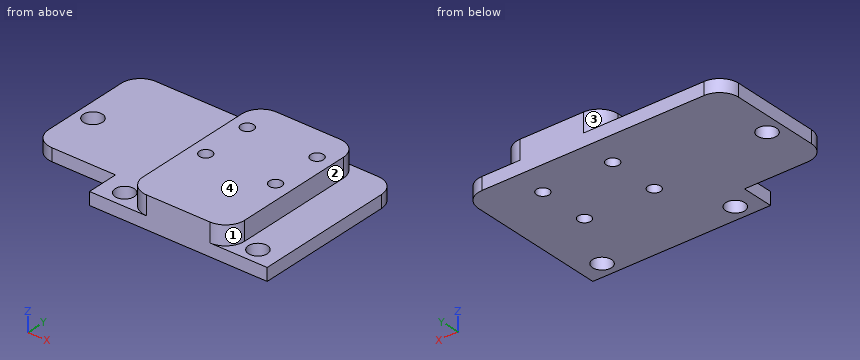
from build123d import *

# Parameters (mm, degrees)
BOSS_EXTRU_1_DEPTH      = 2
ESQUISSE2_W             = 16
ESQUISSE2_H             = 25
BOSS_EXTRU_2_DEPTH      = 3
ENL_V_MAT_EXTRU_1_REACH = 4
ESQUISSE3_R             = 1.5
ENL_V_MAT_EXTRU_2_REACH = 7
ESQUISSE4_R             = 1
ENL_V_MAT_EXTRU_3_REACH = 4
ESQUISSE5_W             = 13
ESQUISSE5_H             = 20
CONG_1_R                = 3


with BuildPart() as part:
    # Esquisse1 → Boss.-Extru.1 (new body)
    with BuildSketch(Plane.XY):
        Polygon((-27, 25), (27, 25), (27, 5), (14, 5), (14, 0), (-14, 0), (-14, 5), (-27, 5), align=None)
    extrude(amount=BOSS_EXTRU_1_DEPTH)

    # Esquisse2 → Boss.-Extru.2 (add)
    with BuildSketch(Plane.XY.offset(2)):
        with Locations((0, 12.5)):
            Rectangle(ESQUISSE2_W, ESQUISSE2_H)
    extrude(amount=BOSS_EXTRU_2_DEPTH)

    # Esquisse3 → Enlèv. mat.-Extru.1 (cut, up to next)
    with BuildSketch(Plane.XY.offset(2), mode=Mode.PRIVATE) as enl_v_mat_extru_1_sk1:
        with Locations((-24.5, 13.5)):
            Circle(ESQUISSE3_R)
    enl_v_mat_extru_1_tool1 = extrude(enl_v_mat_extru_1_sk1.sketch, amount=-ENL_V_MAT_EXTRU_1_REACH, mode=Mode.PRIVATE) & part.part
    add(enl_v_mat_extru_1_tool1.solids().sort_by_distance((-24.5, 13.5, 2))[0], mode=Mode.SUBTRACT)
    # Esquisse3 → Enlèv. mat.-Extru.1 (cut, up to next)
    with BuildSketch(Plane.XY.offset(2), mode=Mode.PRIVATE) as enl_v_mat_extru_1_sk2:
        with Locations((-10.5, 2.5)):
            Circle(ESQUISSE3_R)
    enl_v_mat_extru_1_tool2 = extrude(enl_v_mat_extru_1_sk2.sketch, amount=-ENL_V_MAT_EXTRU_1_REACH, mode=Mode.PRIVATE) & part.part
    add(enl_v_mat_extru_1_tool2.solids().sort_by_distance((-10.5, 2.5, 2))[0], mode=Mode.SUBTRACT)
    # Esquisse3 → Enlèv. mat.-Extru.1 (cut, up to next)
    with BuildSketch(Plane.XY.offset(2), mode=Mode.PRIVATE) as enl_v_mat_extru_1_sk3:
        with Locations((10.5, 2.5)):
            Circle(ESQUISSE3_R)
    enl_v_mat_extru_1_tool3 = extrude(enl_v_mat_extru_1_sk3.sketch, amount=-ENL_V_MAT_EXTRU_1_REACH, mode=Mode.PRIVATE) & part.part
    add(enl_v_mat_extru_1_tool3.solids().sort_by_distance((10.5, 2.5, 2))[0], mode=Mode.SUBTRACT)

    # Esquisse4 → Enlèv. mat.-Extru.2 (cut, up to next)
    with BuildSketch(Plane.XY.offset(5), mode=Mode.PRIVATE) as enl_v_mat_extru_2_sk1:
        with Locations((-5.5, 20)):
            Circle(ESQUISSE4_R)
    enl_v_mat_extru_2_tool1 = extrude(enl_v_mat_extru_2_sk1.sketch, amount=-ENL_V_MAT_EXTRU_2_REACH, mode=Mode.PRIVATE) & part.part
    add(enl_v_mat_extru_2_tool1.solids().sort_by_distance((-5.5, 20, 5))[0], mode=Mode.SUBTRACT)
    # Esquisse4 → Enlèv. mat.-Extru.2 (cut, up to next)
    with BuildSketch(Plane.XY.offset(5), mode=Mode.PRIVATE) as enl_v_mat_extru_2_sk2:
        with Locations((-5.5, 12)):
            Circle(ESQUISSE4_R)
    enl_v_mat_extru_2_tool2 = extrude(enl_v_mat_extru_2_sk2.sketch, amount=-ENL_V_MAT_EXTRU_2_REACH, mode=Mode.PRIVATE) & part.part
    add(enl_v_mat_extru_2_tool2.solids().sort_by_distance((-5.5, 12, 5))[0], mode=Mode.SUBTRACT)
    # Esquisse4 → Enlèv. mat.-Extru.2 (cut, up to next)
    with BuildSketch(Plane.XY.offset(5), mode=Mode.PRIVATE) as enl_v_mat_extru_2_sk3:
        with Locations((5.5, 12)):
            Circle(ESQUISSE4_R)
    enl_v_mat_extru_2_tool3 = extrude(enl_v_mat_extru_2_sk3.sketch, amount=-ENL_V_MAT_EXTRU_2_REACH, mode=Mode.PRIVATE) & part.part
    add(enl_v_mat_extru_2_tool3.solids().sort_by_distance((5.5, 12, 5))[0], mode=Mode.SUBTRACT)
    # Esquisse4 → Enlèv. mat.-Extru.2 (cut, up to next)
    with BuildSketch(Plane.XY.offset(5), mode=Mode.PRIVATE) as enl_v_mat_extru_2_sk4:
        with Locations((5.5, 20)):
            Circle(ESQUISSE4_R)
    enl_v_mat_extru_2_tool4 = extrude(enl_v_mat_extru_2_sk4.sketch, amount=-ENL_V_MAT_EXTRU_2_REACH, mode=Mode.PRIVATE) & part.part
    add(enl_v_mat_extru_2_tool4.solids().sort_by_distance((5.5, 20, 5))[0], mode=Mode.SUBTRACT)

    # Esquisse5 → Enlèv. mat.-Extru.3 (cut, up to next)
    with BuildSketch(Plane.XY.offset(2), mode=Mode.PRIVATE) as enl_v_mat_extru_3_sk1:
        with Locations((20.5, 15)):
            Rectangle(ESQUISSE5_W, ESQUISSE5_H)
    enl_v_mat_extru_3_tool1 = extrude(enl_v_mat_extru_3_sk1.sketch, amount=-ENL_V_MAT_EXTRU_3_REACH, mode=Mode.PRIVATE) & part.part
    add(enl_v_mat_extru_3_tool1.solids().sort_by_distance((20.5, 15, 2))[0], mode=Mode.SUBTRACT)

    # Congé1
    cong_1_edges = [part.edges().sort_by_distance(p)[0] for p in [
        (8, 0, 3.5),
        (-8, 0, 3.5),
        (8, 25, 3.5),
        (-8, 25, 3.5),
        (-27, 5, 1),
        (-27, 25, 1),
        (14, 25, 1),
    ]]
    fillet(cong_1_edges, radius=CONG_1_R)


solid = part.part
Verification items for the finished model (mm, model axes). Face numbers are marked on the shaded views. A direction names the side the tool comes from. Coordinates: 2 decimals unless noted, no trailing zeros. Order: outer loops, then holes, each group sorted by start corner. A loop starts at its lowest first (then second) coordinate and runs counter-clockwise, first axis right, second up.
Item 1: Section check B-B, the plane x = 10.5. Enter the section's corners in (y, z).
Filled in:
outline: (0, 0) - (1, 0) - (1, 2) - (0, 2) - close; (4, 0) - (25, 0) - (25, 2) - (4, 2) - close
Item 2: Depth check by flat-ended pin: pin 1 (2.5 mm diameter, centred on x = -5.5, y = 12, fed in from -Z); pin 2 (2 mm diameter, centred on y = 1.5, z = 0.5, fed in from -X); pin 3 (4 mm diameter, centred on x = -16, y = 21, fed in from +Z); pin 4 (2 mm diameter, centred on x = -16.5, z = 0.5, fed in from -Y). Enter the tip coordinate at first touch or a pass-through.
Filled in:
pin 1: stops at z = 0
pin 2: stops at x = -14
pin 3: stops at z = 2
pin 4: stops at y = 5
Item 3: Section check D-D, the plane z = 1.5. Enter the section's corners in (x, y).
Filled in:
outline: (-27, 8) arc R3 ccw to (-24, 5) - (-14, 5) - (-14, 0) - (14, 0) - (14, 22) arc R3 ccw to (11, 25) - (-24, 25) arc R3 ccw to (-27, 22) - close; hole circle Ø3 at (-24.5, 13.5); hole circle Ø3 at (-10.5, 2.5); hole circle Ø2 at (-5.5, 12); hole circle Ø2 at (-5.5, 20); hole circle Ø2 at (5.5, 12); hole circle Ø2 at (5.5, 20); hole circle Ø3 at (10.5, 2.5)
Item 4: Section check C-C, the plane y = 20. Enter the section's corners in (x, z), then the cut area to 3 significant figures.
Filled in:
outline: (-27, 0) - (-6.5, 0) - (-6.5, 5) - (-8, 5) - (-8, 2) - (-27, 2) - close; (-4.5, 0) - (4.5, 0) - (4.5, 5) - (-4.5, 5) - close; (6.5, 0) - (14, 0) - (14, 2) - (8, 2) - (8, 5) - (6.5, 5) - close
area: 110 mm2
Item 5: Access from +Z, -Z, +X, -X, +Y, -Y to the whole of each face (thin tool, end or side, straight path). Record for the marked faces 1, 2, 3 and 4.
Filled in:
face 1: +Z, +X, -Y
face 2: +Z, +X, +Y, -Y
face 3: +Z, -X, +Y
face 4: +Z, +X, -X, +Y, -Y
Item 6: Section check A-A, the plane y = 13.5. Enter the section's corners in (x, z), then the cut area to 3 significant figures.
Filled in:
outline: (-27, 0) - (-26, 0) - (-26, 2) - (-27, 2) - close; (-23, 0) - (14, 0) - (14, 2) - (8, 2) - (8, 5) - (-8, 5) - (-8, 2) - (-23, 2) - close
area: 124 mm2
Item 7: Material ranges on L1, parallel to Y at x = 5.5, z = 1.4; L2, parallel to X at y = 12.75, z = 3.75; L3, parallel to Z at x = -13.5, y = 10.5, recorded low to high.
Filled in:
L1: y = 0 to 11, 13 to 19, 21 to 25
L2: x = -8 to -6.16, -4.84 to 4.84, 6.16 to 8
L3: z = 0 to 2
